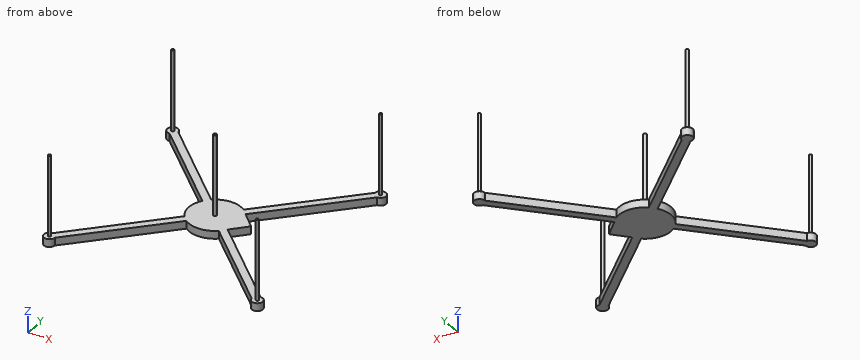
```python
from build123d import *

# Parameters (mm, degrees)
BOSS_EXTRUDE1_DEPTH = 10
SKETCH3_R           = 1.796885627
SKETCH3_R_2         = 2.038704301
BOSS_EXTRUDE2_DEPTH = 113


with BuildPart() as part:
    # Sketch2 → Boss-Extrude1 (new body)
    with BuildSketch(Plane.XY):
        with BuildLine():
            Line((-20.72228509, 26.381237071), (-125.55357923, 131.212531212))
            ThreePointArc((-125.55357923, 131.212531212), (-137.769587184, 135.843703419), (-132.41170091, 123.928517268))
            Line((-132.41170091, 123.928517268), (-27.580406769, 19.097223127))
            ThreePointArc((-27.580406769, 19.097223127), (-33.546725157, 0), (-27.580406769, -19.097223127))
            Line((-27.580406769, -19.097223127), (-132.41170091, -123.928517268))
            ThreePointArc((-132.41170091, -123.928517268), (-137.769587184, -135.843703419), (-125.55357923, -131.212531212))
            Line((-125.55357923, -131.212531212), (-20.72228509, -26.381237071))
            ThreePointArc((-20.72228509, -26.381237071), (0, -33.546725157), (20.72228509, -26.381237071))
            Line((20.72228509, -26.381237071), (125.55357923, -131.212531212))
            ThreePointArc((125.55357923, -131.212531212), (137.769587184, -135.843703419), (132.41170091, -123.928517268))
            Line((132.41170091, -123.928517268), (27.580406769, -19.097223127))
            Line((27.580406769, -19.097223127), (46.005003751, 0))
            Line((46.005003751, 0), (27.580406769, 19.097223127))
            Line((27.580406769, 19.097223127), (132.41170091, 123.928517268))
            ThreePointArc((132.41170091, 123.928517268), (137.769587184, 135.843703419), (125.55357923, 131.212531212))
            Line((125.55357923, 131.212531212), (20.72228509, 26.381237071))
            ThreePointArc((20.72228509, 26.381237071), (0, 33.546725157), (-20.72228509, 26.381237071))
        make_face()
    extrude(amount=BOSS_EXTRUDE1_DEPTH)

    # Sketch3 → Boss-Extrude2 (add)
    with BuildSketch(Plane.XY):
        with Locations((-132.621345525, 130.996476601)):
            Circle(SKETCH3_R)
        with Locations(Location((132.621345525, 130.996476601, 0), (0, 0, 180))):
            Circle(SKETCH3_R)
        with Locations((132.621345525, -130.996476601)):
            Circle(SKETCH3_R)
        with Locations(Location((-132.621345525, -130.996476601, 0), (0, 0, 180))):
            Circle(SKETCH3_R)
        Circle(SKETCH3_R_2)
    extrude(amount=BOSS_EXTRUDE2_DEPTH)


solid = part.part
```
Here's how the part is built. I have some questions about the finished solid (model axes, mm). Coordinates: 2 decimals unless noted, no trailing zeros. Order: outer loops, then holes, each group sorted by start corner. A loop starts at its lowest first (then second) coordinate and runs counter-clockwise, first axis right, second up. Notation, with made-up numbers: (73, 87.5) - (96, 87.5) arc R12 cw to (96, 92.5) - close; hole circle Ø11 at (-4, 43.25). An arc over 180 degrees is marked (long way). One line per question, with ' | ' between items.
(1) Suppose I cut it at D-D on y = -15. List the corners of the cut face in (x, z) for me, and give its area (3 significant figures).
Report:
outline: (-30.01, 0) - (31.53, 0) - (31.53, 10) - (-30.01, 10) - close | area: 615 mm2
(2) Suppose I cut it at A-A on x = 81. List the corners of the cut face in (y, z) for me.
Report:
outline: (-86.66, 0) - (-72.52, 0) - (-72.52, 10) - (-86.66, 10) - close; (72.52, 0) - (86.66, 0) - (86.66, 10) - (72.52, 10) - close
(3) Suppose I cut it at B-B on y = -59. List the corners of the cut face in (x, z) for me, and give its area (3 significant figures).
Report:
outline: (-67.48, 0) - (-53.34, 0) - (-53.34, 10) - (-67.48, 10) - close; (53.34, 0) - (67.48, 0) - (67.48, 10) - (53.34, 10) - close | area: 283 mm2
(4) Suppose I cut it at C-C on z = 22.5. List the corners of the cut face in (x, y) for me.
Report:
outline: circle Ø3.59 at (-132.62, -131); circle Ø3.59 at (-132.62, 131); circle Ø4.08 at (0, 0); circle Ø3.59 at (132.62, -131); circle Ø3.59 at (132.62, 131)
(5) If I drill on L1, parallel to X at y = 119.5, z = 8; L2, parallel to Z at x = -52, y = 55; L3, parallel to Y at x = 126.5, z = 7.5, over which ranges is the centre line in solid material (lowest first)?
Report:
L1: x = -127.98 to -113.84, 113.84 to 127.98 | L2: z = 0 to 10 | L3: y = -134.54 to -118.02, 118.02 to 134.54
